from build123d import *

# Parameters (mm, degrees)
SKETCH1_R      = 4.7625
EXTRUDE1_DEPTH = 3.175


with BuildPart() as part:
    # Sketch1 → Extrude1 (new body)
    with BuildSketch(Plane(origin=(0, 0, 0), x_dir=(1, 0, 0), z_dir=(0, 1, 0))):
        with BuildLine():
            Line((-53.17019082, 56.796126628), (-114.3, 56.796126628))
            Line((-114.3, 56.796126628), (-114.3, 106.008626628))
            Line((-114.3, 106.008626628), (-68.825107544, 106.008626628))
            ThreePointArc((-68.825107544, 106.008626628), (-67.102021241, 106.246877812), (-65.508234891, 106.943753056))
            ThreePointArc((-65.508234891, 106.943753056), (0, 125.4125), (65.508234891, 106.943753056))
            ThreePointArc((65.508234891, 106.943753056), (67.102021241, 106.246877812), (68.825107544, 106.008626628))
            Line((68.825107544, 106.008626628), (114.3, 106.008626628))
            Line((114.3, 106.008626628), (114.3, 56.796126628))
            Line((114.3, 56.796126628), (53.17019082, 56.796126628))
            ThreePointArc((53.17019082, 56.796126628), (50.99326112, 57.180937857), (49.080176141, 58.288732272))
            ThreePointArc((49.080176141, 58.288732272), (0, 76.2), (-49.080176141, 58.288732272))
            ThreePointArc((-49.080176141, 58.288732272), (-50.99326112, 57.180937857), (-53.17019082, 56.796126628))
        make_face()
        with Locations((101.6, 81.402376628)):
            Circle(SKETCH1_R, mode=Mode.SUBTRACT)
        with Locations((-101.6, 81.402376628)):
            Circle(SKETCH1_R, mode=Mode.SUBTRACT)
    extrude(amount=EXTRUDE1_DEPTH)


solid = part.part
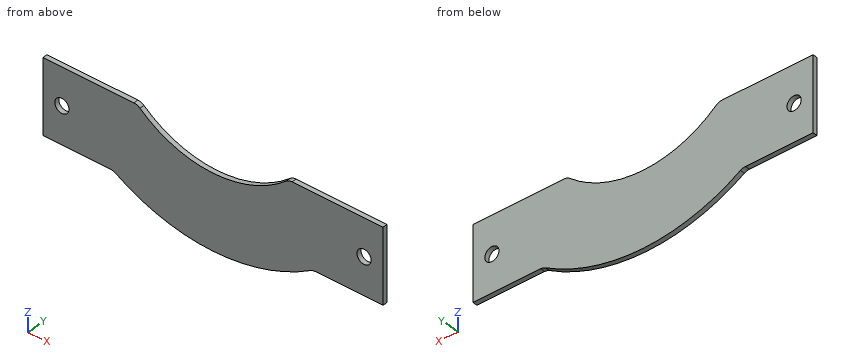
Work out the finished part from the listing and answer in its coordinate system (mm). Round coordinates to 2 decimals unless told otherwise and drop trailing zeros. Write each loop counter-clockwise with the first axis right and the second up, starting at its lowest first coordinate (ties: lowest second). Pieces come first, ordered by that corner, then holes.
1) A cutting plane is placed at D-D (x = 73.5). Give the vertices of the cut face in (y, z) (3 decimals), plus the area to 3 significant figures.
2) A cutting plane is placed at A-A (x = 101.6). Give the vertices of the cut face in (y, z) (3 decimals), plus the area to 3 significant figures.
3) Given pin 1 Ø15 at (x, z) = (101.6, -81.4) entering from +Y (3 decimals); pin 2 Ø10 at (x, z) = (17.5, -66.5) entering from +Y (3 decimals); pin 3 Ø1.6 at (x, y) = (99, 1.5) entering from -Z; pin 4 Ø1 at (x, y) = (45, 2.5) entering from +Z, each flat-ended and moving along its own axis, determine where each tip first touches the part or whether it passes through.
4) A cutting plane is placed at C-C (y = 1.6). Give the number of separate pieces and of enclosed holes in the cut face, plus the area to 3 significant figures.
5) A cutting plane is placed at B-B (z = -63). Give the vertices of the cut face in (x, y) (3 decimals), plus the area to 3 significant figures.
6) Straight lines are drawn through the part: line 1 (X direction, y = 1.05, z = -79.5); line 2 (X direction, y = 2.3, z = -84.5); line 3 (Z direction, x = 101.6, y = 1.6). For each, find the intervals that lie inside material, in ascending order.
Completed:
1. outline: (0, -106.009) - (3.175, -106.009) - (3.175, -56.796) - (0, -56.796) - close
1. area: 156 mm2
2. outline: (0, -106.009) - (3.175, -106.009) - (3.175, -86.165) - (0, -86.165) - close; (0, -76.64) - (3.175, -76.64) - (3.175, -56.796) - (0, -56.796) - close
2. area: 126 mm2
3. pin 1: stops at y = 3.175
3. pin 2: passes through
3. pin 3: stops at z = -106.01
3. pin 4: stops at z = -61.12
4. separate pieces: 1
4. enclosed holes: 2
4. area: 11,500 mm2
5. outline: (-114.3, 0) - (-42.865, 0) - (-42.865, 3.175) - (-114.3, 3.175) - close; (42.865, 0) - (114.3, 0) - (114.3, 3.175) - (42.865, 3.175) - close
5. area: 454 mm2
6. line 1: x = -114.3 to -105.97, -97.23 to 97.23, 105.97 to 114.3
6. line 2: x = -114.3 to -105.22, -97.98 to 97.98, 105.22 to 114.3
6. line 3: z = -106.01 to -86.16, -76.64 to -56.8
